Design review of the part built by this model. Coordinates are the model's own, in mm. Face numbers are marked on the shaded views. Give positions to 0.01 mm unless a question says otherwise; leave off trailing zeros. Loops run counter-clockwise (first coordinate to the right, second up) from the corner with the lowest first, then second, coordinate; pieces in that order, holes last. Notation, with made-up numbers: M 62.25,-17.5 L 95.25,-17.5 A20 ccw 95.25,-12.5 Z; hole C -9,-35.75 d5. An arc over 180 degrees is marked long. Use a Markdown table: item, result. Add a question column.
(1) Insertion check: pin 1 Ø10 at (y, z) = (-6.5, 100.5) entering from -X; pin 2 Ø5 at (x, y) = (-5.5, -17.5) entering from +Z; pin 3 Ø7.5 at (x, y) = (36, -14) entering from +Z. Each pin has a flat end and moves straight along its axis. Give the tip position at first contact, or say it passes through.
(2) Draft analysis for pull direction X (two halves, no side actions). For the marked faces 1, 2 and 3, state which applies: pulls with the +X half, pulls with the -X half, needs draft (parallel to the pull), parting line crosses it, or undercut.
(3) Add section B-B, the plane y = -10.5. State how many separate pieces and enclosed holes the cut face has, then the cut area to 3 significant figures.
(4) Add section A-A, the plane x = 112. Give the boundary of the cut face in (y, z) (3 decimals).
(5) Add section C-C, the plane z = 212. Give the boundary of the cut face in (x, y), then the cut area to 3 significant figures.
(6) Add section D-D, the plane z = 57. Give the boundary of the cut face in (x, y).
(7) For probe 1 along X at (y, z) = (-13.5, 85); probe 2 along X at (y, z) = (-4.25, 128); probe 3 along X at (y, z) = (-10.5, 201), list the stretches that pass through material, from the lowest coordinate up.
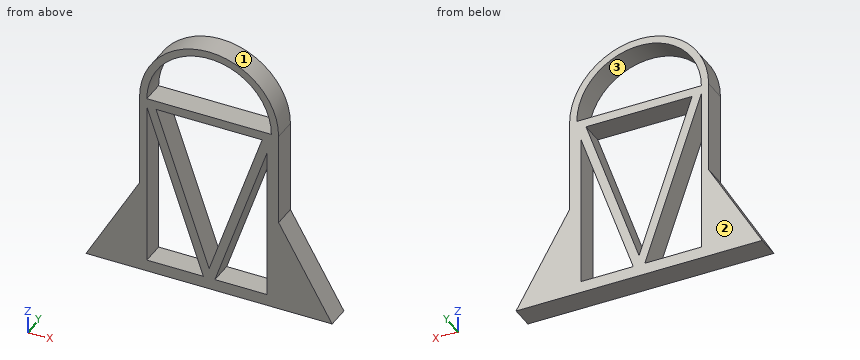
```python
from build123d import *

# Parameters (mm, degrees)
F1_DEPTH = 25.4
F3_DEPTH = 25.401
F5_DEPTH = 25.4


with BuildPart() as f1:
    # F0 (on Front) → F1 (new body)
    with BuildSketch(Plane.XZ):
        with BuildLine():
            Line((0, 203.2), (0, 0))
            Line((0, 0), (152.4, 0))
            Line((152.4, 0), (152.4, 203.2))
            ThreePointArc((152.4, 203.2), (76.2, 279.4), (0, 203.2))
        make_face()
        with BuildLine():
            ThreePointArc((7.9375, 203.2), (76.2, 271.4625), (144.4625, 203.2))
            Line((144.4625, 203.2), (7.9375, 203.2))
        make_face(mode=Mode.SUBTRACT)
    extrude(amount=F1_DEPTH)

    # F2 (on face) → F3 (cut, through all)
    with BuildSketch(Plane.XZ.offset(25.4)):
        Polygon((7.9375, 193.675), (7.9375, 12.7), (69.85, 12.7), align=None)
        Polygon((139.7, 12.7), (139.7, 179.753846), (82.55, 12.7), align=None)
        Polygon((134.395535, 193.675), (18.004465, 193.675), (76.2, 23.564975), align=None)
    extrude(amount=-F3_DEPTH, mode=Mode.SUBTRACT)

    # F4 (on face) → F5 (join, through all)
    with BuildSketch(Plane.XZ.offset(25.4)):
        Polygon((0, 0), (0, 101.6), (-58.658787, 0), align=None)
        Polygon((211.058787, 0), (152.4, 101.6), (152.4, 0), align=None)
    extrude(amount=-F5_DEPTH)


solid = f1.part
```
Established:
| question | item | result |
|---|---|---|
| 1 | pin 1 | x = -3.52 |
| 1 | pin 2 | z = 96.4 |
| 1 | pin 3 | z = 270.12 |
| 2 | face 1 | parting line crosses it |
| 2 | face 2 | needs draft |
| 2 | face 3 | undercut |
| 3 | separate pieces | 1 |
| 3 | enclosed holes | 4 |
| 3 | area | 18,500 mm^2 |
| 4 | outline | M -25.4,0 L 0,0 L 0,12.7 L -25.4,12.7 Z; M -25.4,98.785 L 0,98.785 L 0,128.211 L -25.4,128.211 Z; M -25.4,193.675 L 0,193.675 L 0,203.2 L -25.4,203.2 Z; M -25.4,261.322 L 0,261.322 L 0,270.467 L -25.4,270.467 Z |
| 5 | outline | M 0.51,-25.4 L 8.51,-25.4 L 8.51,0 L 0.51,0 Z; M 143.89,-25.4 L 151.89,-25.4 L 151.89,0 L 143.89,0 Z |
| 5 | area | 406 mm^2 |
| 6 | outline | M -25.75,-25.4 L 7.94,-25.4 L 7.94,0 L -25.75,0 Z; M 54.69,-25.4 L 64.76,-25.4 L 64.76,0 L 54.69,0 Z; M 87.64,-25.4 L 97.71,-25.4 L 97.71,0 L 87.64,0 Z; M 139.7,-25.4 L 178.15,-25.4 L 178.15,0 L 139.7,0 Z |
| 7 | probe 1 | -9.58 to 7.94, 45.12 to 55.18, 97.22 to 107.28, 139.7 to 161.98 |
| 7 | probe 2 | 0 to 7.94, 30.41 to 40.47, 111.93 to 121.99, 139.7 to 152.4 |
| 7 | probe 3 | 0 to 152.4 |
